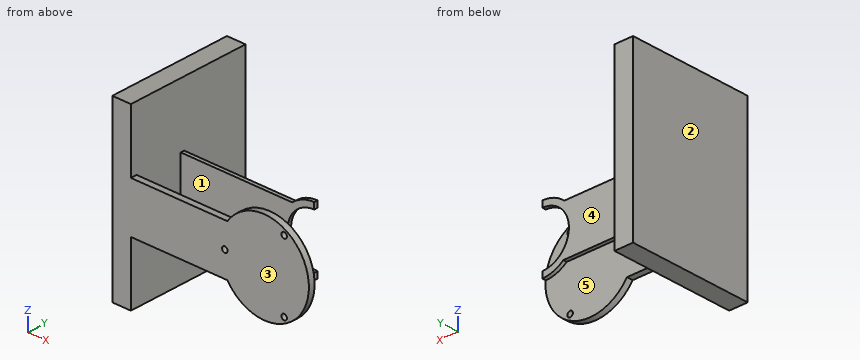
Autodesk Fusion 360 part; units mm, degrees
sketch "스케치1" plane through (0, 0, 0) normal (0, 1, 0) x (1, 0, 0)
  circle A0 centre (0, 0) radius 36
  line L0 (-32.5898, 56.4472) -> (34.7247, -60.145) construction
  line L1 (0, 75) -> (0, -75) construction
  line L2 (51.4685, 0) -> (-45, 0) construction
  line L3 (30.2625, 52.4162) -> (-30.7015, -53.1766) construction
  circle A1 centre (0, 0) radius 32 construction
  circle A2 centre (16, -27.7128) radius 2.25
  circle A3 centre (16, 27.7128) radius 2.25
  circle A4 centre (-32, 0) radius 2.25
  curve L4 construction
  point P0 (16, -27.7128)
  point P1 (16, 27.7128)
  point P2 (-32, 0)
  dimension "d2" = 72
  dimension "d3" = 30
  dimension "d4" = 30
  dimension "d5" = 64
  dimension "d6" = 4.5
  dimension "d29" = 100
extrude "돌출1" add sketch "스케치1" along normal blind 2
extrude "돌출2" add 1 faces at (0, 2, 0) along direction (0, 1, 0) blind 3
sketch "스케치2" plane through (0, 0, 0) normal (0, 1, 0) x (1, 0, 0)
  line L0 (20, -20) -> (-108, -20)
  line L1 (-108, -20) -> (-108, 20)
  line L2 (-108, 20) -> (20, 20)
  line L3 (20, 20) -> (20, -20)
  line L4 (0, 75) -> (0, -75)
  circle A0 centre (0, 0) radius 36
  line L5 (-108, -70) -> (-123, -70)
  line L6 (-123, -70) -> (-123, 70)
  line L7 (-123, 70) -> (-108, 70)
  line L8 (-108, 70) -> (-108, -70)
  dimension "d13" = 40
  dimension "d15" = 20
  dimension "d16" = 108
  dimension "d17" = 50
  dimension "d18" = 50
  dimension "d19" = 15
extrude "돌출3" add sketch "스케치2" along normal blind 5 contours L0 L1 L2 A0 L8 | L1 L5 L6 L7 L8
extrude "돌출4" add sketch "스케치2" along normal blind 10 contours L1 L5 L6 L7 L8
extrude "돌출5" add 1 faces at (-113, 10, 23.3333) along direction (0, 1, 0) blind 15
extrude "돌출6" add 1 faces at (-113, 25, 23.3333) along direction (0, 1, 0) blind 75
ref_plane "작업 평면1" through (-43.5, 45, 0) normal (0, 1, 0) x (1, 0, 0)
sketch "스케치3" plane through (-36, 45, 0) normal (0, 1, 0) x (1, 0, 0)
  arc A0 (36, 21.5) -> (36, -21.5) centre (36, 0) ccw
  curve L0
  arc A1 (36, 26.5) -> (36, -26.5) centre (36, 0) ccw
  line L1 (36, 21.5) -> (36, 26.5)
  line L2 (36, -26.5) -> (36, -21.5)
  dimension "d30" = 21.5
  dimension "d31" = 5
sketch "스케치5" plane through (-36, 45, 0) normal (0, 1, 0) x (1, 0, 0)
  line L0 (19.0243, 20.3488) -> (-72.2102, 20.3488)
  line L1 (-72.2102, 20.3488) -> (-72.2102, -19.6512)
  line L2 (-72.2102, -19.6512) -> (19.0243, -19.6512)
  arc A0 (36, 26.5) -> (36, -26.5) centre (36, 0) ccw
  curve L3
extrude "돌출7" add sketch "스케치3" sketch "스케치5" along normal blind 1.5 of sketch 2
extrude "돌출8" add 1 faces at (-79.1466, 45, -0.7681) along direction (0, -1, 0) blind 1.5
equation "d16 = 72 mm + 36 mm"
equation "d30 = ( 43 / 2 ) * 1 mm"
Can you work these out from the model? Positions are in its coordinate system, mm. Face numbers are marked on the shaded views. A direction names the side the tool comes from. Coordinates: 2 decimals unless noted, no trailing zeros. Loops run counter-clockwise (first coordinate to the right, second up) from the corner with the lowest first, then second, coordinate; pieces in that order, holes last. Notation, with made-up numbers: (-35, -13.5) -> (-29, -13.5) arc R29 ccw to (-29, 20.5) -> close; hole circle Ø10 at (32, 1.5). An arc over 180 degrees is marked (long way). Put each result on its own line as item: value. Start each with the question number.
Q1. I want a section at C-C (x = 16). Write out the boundary of the cut face in (y, z).
Q2. I want a section at D-D (z = 55). Write out the boundary of the cut face in (x, y).
Q3. If I drill on line 1 (Z direction, x = 16, y = 4); line 2 (Y direction, x = -41, z = 0); line 3 (X direction, y = 2, z = 0), over which ranges is the centre line in solid material (lowest first)? Write a range as [from, to].
Q4. I'm going to push flat-ended pins straight in: P1, Ø4, axis at x = -56.5, y = 2, coming from the -Z side; P2, Ø1.5, axis at x = -58, y = 3, coming from the +Z side; P3, Ø2.5, axis at y = 45.5, z = -23, coming from the +X side. Where does each tip first touch, or does it pass through?
Q5. I want a section at B-B (z = 0). Write out the boundary of the cut face in (x, y), plus the area to 3 significant figures.
Q6. For the marked faces 1 and 2, which set-ups out of +Z, -Z, +X, -X, +Y, -Y let a thin tool reach every point of the face, with its end or its side?
Q7. Thinking about a two-plate mould opening in Y: for the marked faces 3, 4 and 5, which applies, pulls with the +Y half, pulls with the -Y half, needs draft (parallel to the pull), parting line crosses it, or undercut?
Q8. I want a section at A-A (x = -101.5). Write out the boundary of the cut face in (y, z).
Taken from the geometry:
1. outline: (0, -32.25) -> (5, -32.25) -> (5, -29.96) -> (0, -29.96) -> close; (0, -25.46) -> (5, -25.46) -> (5, 25.46) -> (0, 25.46) -> close; (0, 29.96) -> (5, 29.96) -> (5, 32.25) -> (0, 32.25) -> close
2. outline: (-123, 0) -> (-108, 0) -> (-108, 100) -> (-123, 100) -> close
3. line 1: z = [-32.25, -29.96], [-25.46, 25.46], [29.96, 32.25]
3. line 2: y = [0, 5], [43.5, 46.5]
3. line 3: x = [-123, -34.25], [-29.75, 36]
4. P1: stops at z = -20
4. P2: stops at z = 20
4. P3: stops at x = 0
5. outline: (-123, 0) -> (-34.25, 0) -> (-34.25, 5) -> (-108, 5) -> (-108, 43.5) -> (-21.5, 43.5) -> (-21.5, 46.5) -> (-108, 46.5) -> (-108, 100) -> (-123, 100) -> close; (-29.75, 0) -> (36, 0) -> (36, 5) -> (-29.75, 5) -> close
5. area: 2,460 mm2
6. face 1: +Z, -Z, +X
6. face 2: +Z, -Z, -X, +Y, -Y
7. face 3: pulls with the -Y half
7. face 4: pulls with the +Y half
7. face 5: undercut
8. outline: (0, -20) -> (5, -20) -> (5, 20) -> (0, 20) -> close; (43.5, -20.35) -> (46.5, -20.35) -> (46.5, 19.65) -> (43.5, 19.65) -> close
